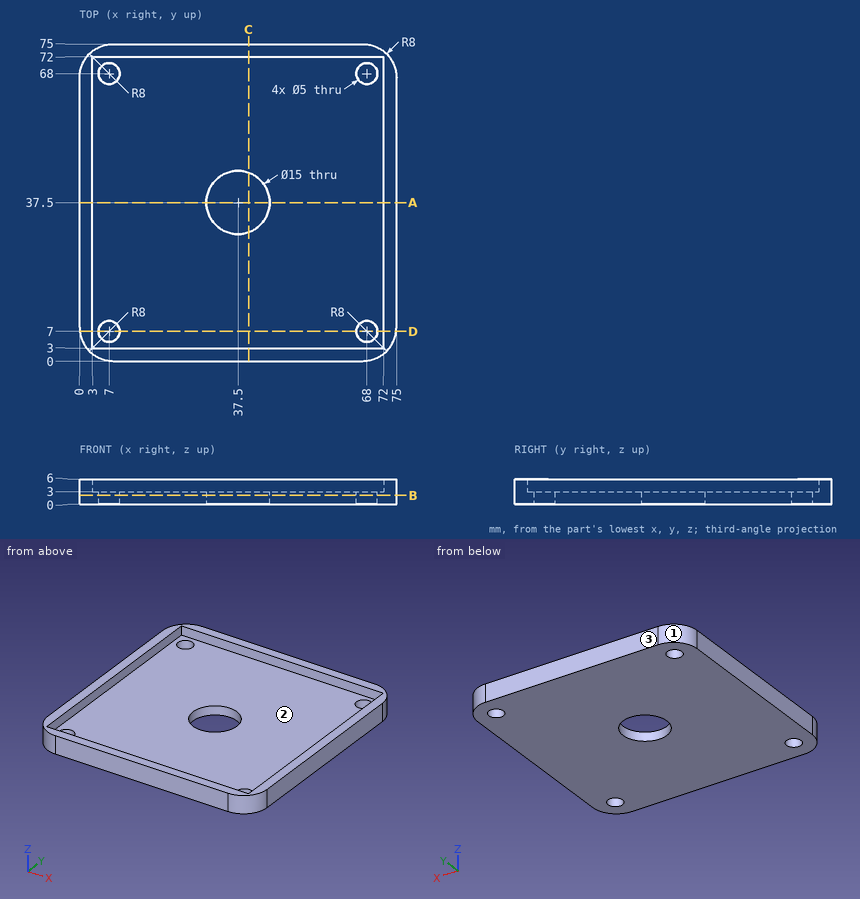
Part print with two shaded views. Sizes in mm from the minimum x, y, z corner. Coordinates: 2 decimals unless noted, no trailing zeros. Order: outer loops, then holes, each group sorted by start corner. A loop starts at its lowest first (then second) coordinate and runs counter-clockwise, first axis right, second up. Notation, with made-up numbers: (-20, -8) - (-12, -8) arc R6 ccw to (-12, 2) - close; hole circle Ø9 at (-38, 12). An arc over 180 degrees is marked (long way). Answer in a Markdown table with one row per item.
1. Slice it at D-D, the plane y = 7. List the corners of the cut face in (x, z).
Answer:
| item | result |
|---|---|
| outline | (0.06, 0) - (4.5, 0) - (4.5, 3) - (3, 3) - (3, 6) - (0.06, 6) - close; (9.5, 0) - (65.5, 0) - (65.5, 3) - (9.5, 3) - close; (70.5, 0) - (74.94, 0) - (74.94, 6) - (72, 6) - (72, 3) - (70.5, 3) - close |
2. Drill centre lines: L1, parallel to Y at x = 18.5, z = 3.95; L2, parallel to Y at x = 7, z = 2. Where is each one in solid material? Low to high. Write a range as from..to.
Answer:
| item | result |
|---|---|
| L1 | 0..3, 72..75 |
| L2 | 0.06..4.5, 9.5..65.5, 70.5..74.94 |
3. Slice it at A-A, the plane y = 37.5. List the corners of the cut face in (x, z).
Answer:
| item | result |
|---|---|
| outline | (0, 0) - (30, 0) - (30, 3) - (3, 3) - (3, 6) - (0, 6) - close; (45, 0) - (75, 0) - (75, 6) - (72, 6) - (72, 3) - (45, 3) - close |
4. Slice it at C-C, the plane x = 40. List the corners of the cut face in (y, z), then the cut area to 3 significant figures.
Answer:
| item | result |
|---|---|
| outline | (0, 0) - (30.43, 0) - (30.43, 3) - (3, 3) - (3, 6) - (0, 6) - close; (44.57, 0) - (75, 0) - (75, 6) - (72, 6) - (72, 3) - (44.57, 3) - close |
| area | 201 mm² |
5. Pull direction X, two halves, no side cores. Call the marked faces 1, 2 and 3: +X half, -X half, draft (parallel to the pull), parting line (faces both ways), or undercut.
Answer:
| item | result |
|---|---|
| face 1 | -X half |
| face 2 | undercut |
| face 3 | draft |
6. Slice it at B-B, the plane z = 2.15. List the corners of the cut face in (x, y), then the cut area to 3 significant figures.
Answer:
| item | result |
|---|---|
| outline | (0, 8) arc R8 ccw to (8, 0) - (67, 0) arc R8 ccw to (75, 8) - (75, 67) arc R8 ccw to (67, 75) - (8, 75) arc R8 ccw to (0, 67) - close; hole circle Ø5 at (7, 7); hole circle Ø5 at (7, 68); hole circle Ø15 at (37.5, 37.5); hole circle Ø5 at (68, 7); hole circle Ø5 at (68, 68) |
| area | 5,310 mm² |
7. Flat gauge pins, fed straight in: P1, Ø12, axis at x = 22.5, y = 52, coming from the +Z side; P2, Ø3, axis at x = 68, y = 7, coming from the -Z side. Where does each tip first touch, or does it go through?
Answer:
| item | result |
|---|---|
| P1 | z = 3 |
| P2 | through |
